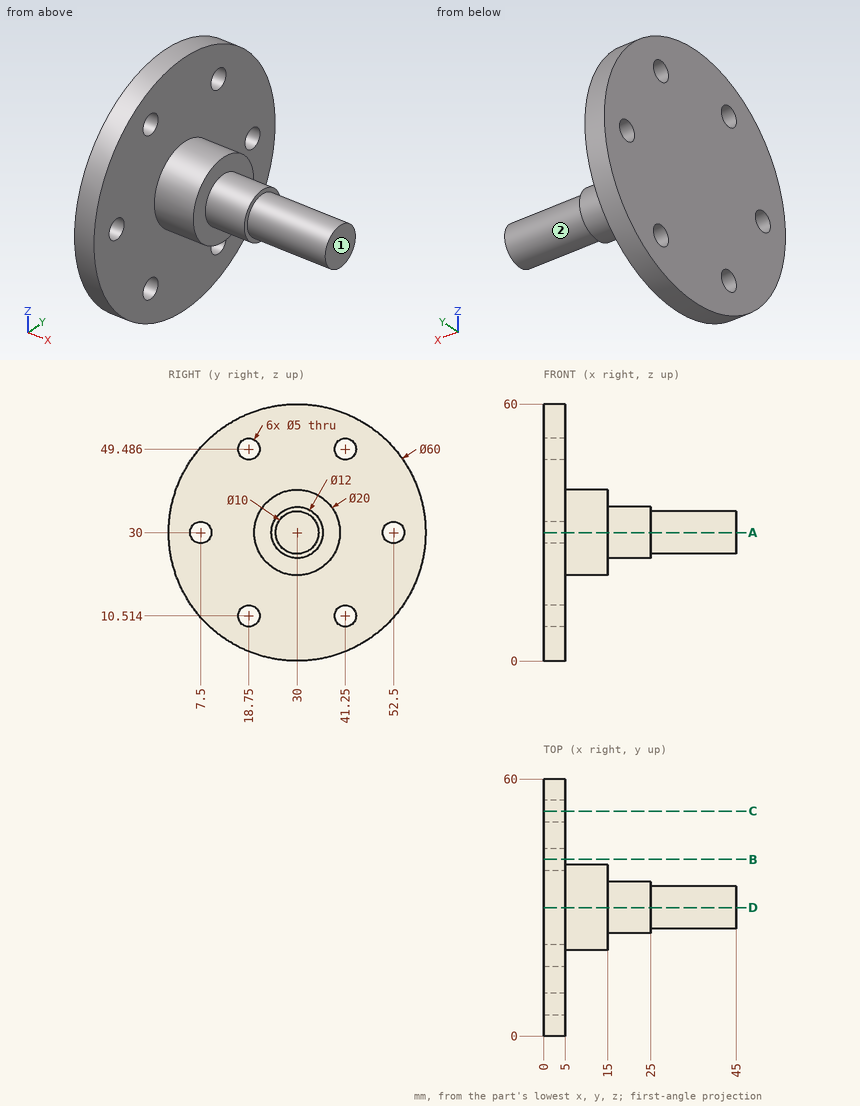
Answer from the drawing. Dimensions are ordinates in mm from the lowest x, y and z of the part. A direction names the side the tool comes from. Coordinates: 2 decimals unless noted, no trailing zeros. Loops run counter-clockwise (first coordinate to the right, second up) from the corner with the lowest first, then second, coordinate; pieces in that order, holes last. Notation, with made-up numbers: (-32, -26) - (-24, -26) arc R30 cw to (-24, -4) - close; hole circle Ø4 at (7, 45). An arc over 180 degrees is marked (long way). Use a Markdown table: item, result.
Item 1: For the marked faces 1 and 2, determine the directions among +Z, -Z, +X, -X, +Y, -Y from which every point of the face is accessible in a straight line to the end or side of a thin tool.
Evaluation:
| item | result |
|---|---|
| face 1 | +Z, -Z, +X, +Y, -Y |
| face 2 | +X |
Item 2: Find section D-D, the plane y = 30. Determine the outline of the cut face in (x, z), and give its area (3 significant figures).
Evaluation:
| item | result |
|---|---|
| outline | (0, 0) - (5, 0) - (5, 20) - (15, 20) - (15, 24) - (25, 24) - (25, 25) - (45, 25) - (45, 35) - (25, 35) - (25, 36) - (15, 36) - (15, 40) - (5, 40) - (5, 60) - (0, 60) - close |
| area | 820 mm2 |
Item 3: Find section B-B, the plane y = 41.25. Determine the outline of the cut face in (x, z) (1 decimal).
Evaluation:
| item | result |
|---|---|
| outline | (0, 2.2) - (5, 2.2) - (5, 8) - (0, 8) - close; (0, 13) - (5, 13) - (5, 47) - (0, 47) - close; (0, 52) - (5, 52) - (5, 57.8) - (0, 57.8) - close |
Item 4: Consider probe 1 along Z at (x, y) = (3, 18) (1 decimal); probe 2 along Z at (x, y) = (3.6, 18.75) (1 decimal); probe 3 along X at (y, z) = (21.5, 28). Determine where each line is inside the solid, lowest interval first. Write a range as from..to.
Evaluation:
| item | result |
|---|---|
| probe 1 | z = 2.5..8.1, 12.9..47.1, 51.9..57.5 |
| probe 2 | z = 2.2..8, 13..47, 52..57.8 |
| probe 3 | x = 0..15 |
Item 5: Find section A-A, the plane z = 30. Determine the outline of the cut face in (x, y).
Evaluation:
| item | result |
|---|---|
| outline | (0, 0) - (5, 0) - (5, 5) - (0, 5) - close; (0, 10) - (5, 10) - (5, 20) - (15, 20) - (15, 24) - (25, 24) - (25, 25) - (45, 25) - (45, 35) - (25, 35) - (25, 36) - (15, 36) - (15, 40) - (5, 40) - (5, 50) - (0, 50) - close; (0, 55) - (5, 55) - (5, 60) - (0, 60) - close |
Item 6: Find section C-C, the plane y = 52.5. Determine the outline of the cut face in (x, z).
Evaluation:
| item | result |
|---|---|
| outline | (0, 10.16) - (5, 10.16) - (5, 27.5) - (0, 27.5) - close; (0, 32.5) - (5, 32.5) - (5, 49.84) - (0, 49.84) - close |
Item 7: Given pin 1 Ø6 at (y, z) = (18.75, 49.49) entering from -X; pin 2 Ø2 at (y, z) = (20, 48.5) entering from +X; pin 3 Ø10 at (x, z) = (40, 19) entering from +Y; pin 4 Ø5 at (x, z) = (29.5, 23.5) entering from +Y, each flat-ended and moving along its own axis, determine where each tip first touches the part or whether it passes through.
Evaluation:
| item | result |
|---|---|
| pin 1 | stops at x = 0 |
| pin 2 | stops at x = 5 |
| pin 3 | passes through |
| pin 4 | stops at y = 33 |
